Read the model definition and answer for the solid it produces. Units are mm, in the model's axes. Face numbers are marked on the shaded views. A direction names the side the tool comes from. Round coordinates to 2 decimals unless told otherwise and drop trailing zeros. Order: outer loops, then holes, each group sorted by start corner. A loop starts at its lowest first (then second) coordinate and runs counter-clockwise, first axis right, second up.
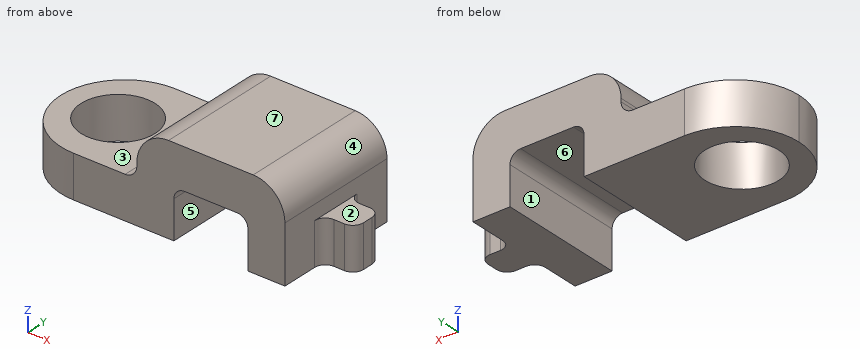
Autodesk Fusion 360 part; units mm, degrees
sketch "Skizze8" plane through (0, 0, 0) normal (0, 1, 0) x (1, 0, 0)
  line L0 (-9.5, 0) -> (-1.75, 0)
  line L1 (-1.75, 0) -> (-1.75, -2.3)
  line L2 (-1.75, -2.3) -> (1.75, -2.3)
  line L3 (1.75, -2.3) -> (1.75, 0)
  line L4 (1.75, 0) -> (3.5, 0)
  line L5 (3.5, -2) -> (3.5, -4.2)
  line L6 (3.5, -4.2) -> (-3.5, -4.2)
  line L7 (-3.5, -4.2) -> (-3.5, -2)
  line L8 (-3.5, -2) -> (-9.5, -2)
  line L9 (-9.5, -2) -> (-9.5, 0)
  line L10 (3.5, 0) -> (5, 0)
  line L11 (5, 0) -> (5, -2)
  line L12 (5, -2) -> (3.5, -2)
  dimension "d100" = 3.5
  dimension "d101" = 1.75
  dimension "d102" = 2.3
  dimension "d103" = 7
  dimension "d104" = 3.5
  dimension "d105" = 4.2
  dimension "d110" = 2
  dimension "d123" = 6
  dimension "d134" = 1.5
extrude "Extrusion5" add sketch "Skizze8" along normal blind 6
sketch "Skizze9" plane through (0, 0, 0) normal (0, 0, 1) x (1, 0, 0)
  line L0 (-9.5, 0) -> (-9.5, 6)
  line L1 (-3.5, 0) -> (-9.5, 0)
  line L2 (-3.5, 0) -> (-3.5, 6)
  line L3 (0, 1.75) -> (0, 22.5)
  point P0 (-6.8, 3)
  point P1 (6.8, 3)
  dimension "d113" = 6
  dimension "d114" = 3
  dimension "d120" = 9.5
  dimension "d128" = 3.3
hole "Bohrung4" at (-6.8, 3, 0) at (6.8, 3, 0) direction (0, 0, 1) diameter 3.5 depth 5 tip angle 118
fillet "Abrundung7" radius 3 2 edges at (-9.5, 0, 1) (-9.5, 6, 1)
fillet "Abrundung8" radius 0.55 1 edges at (-3.5, 3, 2)
fillet "Abrundung9" radius 0.5 2 edges at (-1.75, 3, 2.3) (1.75, 3, 2.3)
fillet "Abrundung10" radius 1.5 2 edges at (-3.5, 3, 4.2) (3.5, 3, 4.2)
sketch "Skizze10" plane through (0, 0, 0) normal (0, 0, 1) x (1, 0, 0)
  line L0 (3.5, 0) -> (5, 0)
  line L1 (5, 0) -> (5, 2.25)
  line L2 (5, 2.25) -> (3.5, 2.25)
  line L3 (3.5, 2.25) -> (3.5, 0)
  line L4 (3.5, 6) -> (5, 6)
  line L5 (5, 6) -> (5, 3.75)
  line L6 (5, 3.75) -> (3.5, 3.75)
  line L7 (3.5, 3.75) -> (3.5, 6)
  line L8 (3.5, 0) -> (5, 0)
  line L9 (5, 0) -> (5, 6)
  line L10 (5, 6) -> (3.5, 6)
  line L11 (3.5, 6) -> (3.5, 0)
  line L12 (3.5, 6) -> (5, 6)
  line L13 (5, 0) -> (3.5, 0)
  dimension "d135" = 1.5
  dimension "d136" = 1.5
  dimension "d141" = 1.5
extrude "Extrusion6" cut sketch "Skizze10" along normal up to surface (2 mm away) contours L0 L1 L2 L3 L8 L9 L11 L13 | L4 L5 L6 L7 L9 L10 L11 L12
fillet "Abrundung11" radius 0.5 4 edges at (3.5, 2.25, 1) (3.5, 3.75, 1) (5, 2.25, 1) (5, 3.75, 1)
equation "d101 = d100 / 2"
equation "d104 = d103 / 2"
equation "d110 = d106"
equation "d114 = d113 / 2"
Q1. A cutting plane is placed at A-A, the plane z = 1.6. Give the number of separate pieces and of enclosed holes in the cut face, plus the area to 3 significant figures.
Outcome:
separate pieces: 2
enclosed holes: 1
area: 45.8 mm2
Q2. A cutting plane is placed at D-D, the plane x = -3.25. Give the vertices of the cut face in (y, z).
Outcome:
outline: (0, 0) - (6, 0) - (6, 3.53) - (0, 3.53) - close
Q3. A cutting plane is placed at B-B, the plane x = -6.8. Give the vertices of the cut face in (y, z), plus the area to 3 significant figures.
Outcome:
outline: (0.01, 0) - (1.25, 0) - (1.25, 2) - (0.01, 2) - close; (4.75, 0) - (5.99, 0) - (5.99, 2) - (4.75, 2) - close
area: 4.94 mm2
Q4. For a pull along X with two mould halves and no side action, classify the marked faces 4, 5, 6 and 7 as released by +X, released by -X, zero draft, split by the parting line, or undercut.
Outcome:
face 4: released by +X
face 5: undercut
face 6: undercut
face 7: zero draft
Q5. For the marked faces 1, 2 and 3, determine the directions among +Z, -Z, +X, -X, +Y, -Y from which every point of the face is accessible in a straight line to the end or side of a thin tool.
Outcome:
face 1: -Z, +Y, -Y
face 2: +Z, +X, +Y, -Y
face 3: +Z, -X, +Y, -Y
Q6. Flat-ended cylindrical pins translate along their axes: pin 1 (1.5 mm diameter, centred on y = 1.5, z = 3, fed in from -X); pin 2 (0.5 mm diameter, centred on y = 4, z = 1, fed in from -X); pin 3 (3 mm diameter, centred on x = 0.5, y = 4, fed in from -Z); pin 4 (0.6 mm diameter, centred on x = 4.5, z = 0.5, fed in from -Y). Find the tip coordinate at first contact, or state that the pin passes through.
Outcome:
pin 1: stops at x = -3.59
pin 2: stops at x = -9.4
pin 3: stops at z = 0
pin 4: stops at y = 2.25
Q7. Straight lines are drawn through the part: probe 1 along X at (y, z) = (3, 0.45); probe 2 along X at (y, z) = (3.85, 0.6); probe 3 along X at (y, z) = (2.15, 2.8). For each, find the intervals that lie inside material, in ascending order.
Outcome:
probe 1: x = -9.5 to -8.55, -5.05 to -1.75, 1.75 to 5
probe 2: x = -9.38 to -8.33, -5.27 to -1.75, 1.75 to 3.7
probe 3: x = -3.5 to 3.5
Q8. A cutting plane is placed at C-C, the plane y = 0.8. Give the vertices of the cut face in (x, z), plus the area to 3 significant figures.
Outcome:
outline: (-8.54, 0) - (-1.75, 0) - (-1.75, 1.8) arc R0.5 cw to (-1.25, 2.3) - (1.25, 2.3) arc R0.5 cw to (1.75, 1.8) - (1.75, 0) - (3.5, 0) - (3.5, 2.7) arc R1.5 ccw to (2, 4.2) - (-2, 4.2) arc R1.5 ccw to (-3.5, 2.7) - (-3.5, 2.55) arc R0.55 cw to (-4.05, 2) - (-8.54, 2) - close
area: 30.6 mm2
